Can you work these out from the model? Positions are in its coordinate system, mm. Face numbers are marked on the shaded views. A direction names the side the tool comes from. Coordinates: 2 decimals unless noted, no trailing zeros. Loops run counter-clockwise (first coordinate to the right, second up) from the corner with the lowest first, then second, coordinate; pieces in that order, holes last. Notation, with made-up numbers: M 7,45 L 18,45 A16 ccw 18,72 Z; hole C -4.5,0 d8. An arc over 180 degrees is marked long. Answer as a JSON object with one key per item and string values. Group by question number.
Item 1: Suppose I cut it at C-C (z = 0.45). Write out the boundary of the cut face in (x, y), then the cut area to 3 significant figures.
Item 2: Suppose I cut it at A-A (y = 17). Write out the boundary of the cut face in (x, z), then the cut area to 3 significant figures.
Item 3: Suppose I cut it at B-B (x = -32). Write out the boundary of the cut face in (y, z).
Item 4: Which directions (+Z, -Z, +X, -X, +Y, -Y) give clear straight access to the entire face, cutting with the end or side of a thin tool? Please do the marked faces 4, 5 and 6.
Item 5: We'd pull the mould along Y, two halves only. Please class the marked faces 1, 2 and 3: +Y half, -Y half, draft (parallel to the pull), parting line (faces both ways), or undercut.
Item 6: Suppose I cut it at D-D (y = 0). Write out the boundary of the cut face in (x, z), then the cut area to 4 significant figures.
Item 7: If I drill on line 1 (Y direction, x = -32, z = 1.6); line 2 (Y direction, x = -25, z = 0.75); line 3 (Y direction, x = -33.25, z = 0.85), over which ranges is the centre line in solid material (lowest first)?
Item 8: I'm going to push a flat-ended pin straight in: pin 1 Ø0.9 at (x, z) = (-27, 2) entering from -Y. Where does the tip first touch, or does it pass through?
```python
from build123d import *

# Parameters (mm, degrees)
SKETCH_R   = 1.6
SKETCH_R_2 = 1.05
PAD_DEPTH  = 3
FILLET_R   = 2.5


with BuildPart() as part:
    # Sketch → Pad (new body)
    with BuildSketch(Plane.XY):
        with BuildLine():
            Line((-35, 20), (-29, 20))
            Line((-29, 20), (-29, 2.05))
            Line((-29, 2.05), (-25, 2.05))
            ThreePointArc((-24.999986, -2.05), (-22.95, 7e-06), (-25, 2.05))
            Line((-24.999986, -2.05), (-29, -2.05))
            Line((-29, -2.05), (-29, -20))
            Line((-29, -20), (-35, -20))
            Line((-35, -20), (-35, 20))
        make_face()
        with Locations((-32, 17)):
            Circle(SKETCH_R, mode=Mode.SUBTRACT)
        with Locations((-32, -17)):
            Circle(SKETCH_R, mode=Mode.SUBTRACT)
        with Locations((-25, 0)):
            Circle(SKETCH_R_2, mode=Mode.SUBTRACT)
    extrude(amount=PAD_DEPTH)

    # Fillet
    fillet_edges = [part.edges().sort_by_distance(p)[0] for p in [
        (-29, -20, 1.5),
        (-35, -20, 1.5),
        (-29, 20, 1.5),
        (-35, 20, 1.5),
    ]]
    fillet(fillet_edges, radius=FILLET_R)


solid = part.part
```
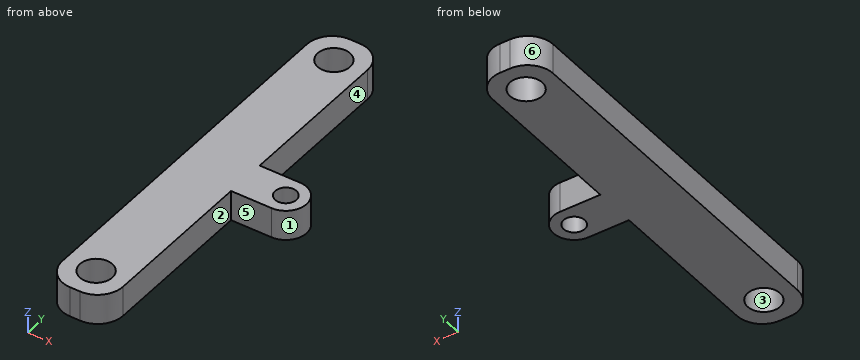
From the geometry:
{
 "1": {"outline": "M -35,-17.5 A2.5 ccw -32.5,-20 L -31.5,-20 A2.5 ccw -29,-17.5 L -29,-2.05 L -25,-2.05 A2.05 ccw -25,2.05 L -29,2.05 L -29,17.5 A2.5 ccw -31.5,20 L -32.5,20 A2.5 ccw -35,17.5 Z; hole C -32,-17 d3.2; hole C -32,17 d3.2; hole C -25,0 d2.1", "area": "238 mm2"},
 "2": {"outline": "M -35,0 L -33.6,0 L -33.6,3 L -35,3 Z; M -30.4,0 L -29,0 L -29,3 L -30.4,3 Z", "area": "8.40 mm2"},
 "3": {"outline": "M -20,0 L -18.6,0 L -18.6,3 L -20,3 Z; M -15.4,0 L 15.4,0 L 15.4,3 L -15.4,3 Z; M 18.6,0 L 20,0 L 20,3 L 18.6,3 Z"},
 "4": {"face 4": "+Z, -Z, +X, +Y", "face 5": "+Z, -Z, +X, -Y", "face 6": "+Z, -Z, -X, +Y"},
 "5": {"face 1": "parting line", "face 2": "draft", "face 3": "undercut"},
 "6": {"outline": "M -35,0 L -26.05,0 L -26.05,3 L -35,3 Z; M -23.95,0 L -22.95,0 L -22.95,3 L -23.95,3 Z", "area": "29.85 mm2"},
 "7": {"line 1": "-20 to -18.6, -15.4 to 15.4, 18.6 to 20", "line 2": "-2.05 to -1.05, 1.05 to 2.05", "line 3": "-19.88 to -18, -16 to 16, 18 to 19.88"},
 "8": {"pin 1": "y = -2.05"}
}
